For this review, take the finished solid that the model builds, in its own axes (mm). Coordinates: 2 decimals unless noted, no trailing zeros. Loops run counter-clockwise (first coordinate to the right, second up) from the corner with the lowest first, then second, coordinate; pieces in that order, holes last. Notation, with made-up numbers: (59.5, 84.25) - (113.5, 84.25) arc R19 ccw to (113.5, 105.25) - close; hole circle Ø6 at (5.5, 46). An arc over 180 degrees is marked (long way). Answer as a JSON object with one key per item and string values. Group by question number.
Item 1: To check wall thickness, follow line 1 (Z direction, x = 0.75, y = -2); line 2 (Y direction, x = 1.25, z = 0.7); line 3 (Y direction, x = 2, z = -0.2). State the ranges of each line that lie inside material, in increasing order.
Item 2: Mouldability with a two-part tool opening along X and no side actions: class faces 1 (the cylindrical face through (-0.07, 57.15, 0)), 2 (the flat face through (0, 1, -0.25)) as released by +X, released by -X, zero draft, split by the parting line, or undercut.
Item 3: We need section C-C (x = 0). Give the boundary of the cut face in (y, z).
Item 4: We need section A-A (z = 0.4). Give the boundary of the cut face in (x, y), then the cut area to 3 significant figures.
Item 5: Clearance check with flat-ended pins moving along their axes: pin 1 (0.6 mm diameter, centred on x = -2, y = -58, fed in from -Z); pin 2 (0.5 mm diameter, centred on x = -1, z = 0, fed in from -Y); pin 3 (1.9 mm diameter, centred on x = 0.5, y = 23, fed in from +Z). State where each tip first meets the part, or that it passes through.
Item 6: We need section B-B (y = 8). Give the boundary of the cut face in (x, z) (3 decimals), then the cut area to 4 significant figures.
from build123d import *

# Parameters (mm, degrees)
RESSALTO_EXTRUS_O1_DEPTH = 0.25
RESSALTO_EXTRUS_O2_DEPTH = 0.5


with BuildPart() as part:
    # Esboço3 → Ressalto-extrusão1 (new, symmetric)
    with BuildSketch(Plane.XY):
        with BuildLine():
            Line((3.175, -57.15), (-3.175, -57.15))
            Line((-3.175, -57.15), (-3.175, 53.975))
            ThreePointArc((-3.175, 53.975), (0, 57.15), (3.175, 53.975))
            Line((3.175, 53.975), (3.175, -57.15))
        make_face()
    extrude(amount=RESSALTO_EXTRUS_O1_DEPTH, both=True)

    # Esboço4 → Ressalto-extrusão2 (add)
    with BuildSketch(Plane.XY.offset(0.25)):
        Polygon((-1.1875, -54.15), (-1.9875, -54.15), (-1.9875, -57.15), (-1.9375, -57.15), (-1.2375, -57.15), (-1.1875, -57.15), align=None)
        with BuildLine():
            Line((-1.2375, -57.15), (-1.9375, -57.15))
            ThreePointArc((-1.9375, -57.15), (-1.831433983, -57.193933983), (-1.7875, -57.3))
            Line((-1.7875, -57.3), (-1.7875, -59.15))
            Line((-1.7875, -59.15), (-1.3875, -59.15))
            Line((-1.3875, -59.15), (-1.3875, -57.3))
            ThreePointArc((-1.3875, -57.3), (-1.343566017, -57.193933983), (-1.2375, -57.15))
        make_face()
    ressalto_extrus_o2 = extrude(amount=RESSALTO_EXTRUS_O2_DEPTH)

    # Espelhar2: Ressalto-extrusão2 across plane
    add(ressalto_extrus_o2.mirror(Plane(origin=(0, 0, 0), x_dir=(0, 0, 1), z_dir=(1, 0, 0))))


solid = part.part
Check sheet entries:
{
 "1": {"line 1": "z = -0.25 to 0.25", "line 2": "y = -57.15 to -54.15", "line 3": "y = -57.15 to 56.44"},
 "2": {"face 1": "split by the parting line", "face 2": "zero draft"},
 "3": {"outline": "(-57.15, -0.25) - (57.15, -0.25) - (57.15, 0.25) - (-57.15, 0.25) - close"},
 "4": {"outline": "(-1.99, -57.15) - (-1.94, -57.15) arc R0.15 cw to (-1.79, -57.3) - (-1.79, -59.15) - (-1.39, -59.15) - (-1.39, -57.3) arc R0.15 cw to (-1.24, -57.15) - (-1.19, -57.15) - (-1.19, -54.15) - (-1.99, -54.15) - close; (1.19, -57.15) - (1.24, -57.15) arc R0.15 cw to (1.39, -57.3) - (1.39, -59.15) - (1.79, -59.15) - (1.79, -57.3) arc R0.15 cw to (1.94, -57.15) - (1.99, -57.15) - (1.99, -54.15) - (1.19, -54.15) - close", "area": "6.42 mm2"},
 "5": {"pin 1": "stops at z = 0.25", "pin 2": "stops at y = -57.15", "pin 3": "stops at z = 0.25"},
 "6": {"outline": "(-3.175, -0.25) - (3.175, -0.25) - (3.175, 0.25) - (-3.175, 0.25) - close", "area": "3.175 mm2"}
}
